```python
from build123d import *

# Parameters (mm, degrees)
BOSS_EXTRUDE1_DEPTH = 21
BOSS_EXTRUDE1_TAPER = 5
SKETCH2_R           = 1.5
CUT_EXTRUDE1_DEPTH  = 10
SKETCH3_R           = 2.75
CUT_EXTRUDE2_DEPTH  = 2


with BuildPart() as part:
    # Sketch1 → Boss-Extrude1 (new body)
    with BuildSketch(Plane.XY):
        with BuildLine():
            Line((-5.5, -7.5), (5.5, -7.5))
            ThreePointArc((5.5, -7.5), (6.914213562, -6.914213562), (7.5, -5.5))
            Line((7.5, -5.5), (7.5, 5.5))
            ThreePointArc((7.5, 5.5), (6.914213562, 6.914213562), (5.5, 7.5))
            Line((5.5, 7.5), (-5.5, 7.5))
            ThreePointArc((-5.5, 7.5), (-6.914213562, 6.914213562), (-7.5, 5.5))
            Line((-7.5, 5.5), (-7.5, -5.5))
            ThreePointArc((-7.5, -5.5), (-6.914213562, -6.914213562), (-5.5, -7.5))
        make_face()
    extrude(amount=BOSS_EXTRUDE1_DEPTH, taper=BOSS_EXTRUDE1_TAPER)

    # Sketch2 → Cut-Extrude1 (cut)
    with BuildSketch(Plane(origin=(0, 0, 0), x_dir=(-1, 0, 0), z_dir=(0, 0, -1))):
        Circle(SKETCH2_R)
    extrude(amount=-CUT_EXTRUDE1_DEPTH, mode=Mode.SUBTRACT)

    # Sketch3 → Cut-Extrude2 (cut)
    with BuildSketch(Plane.XY.offset(21)):
        Circle(SKETCH3_R)
    extrude(amount=-CUT_EXTRUDE2_DEPTH, mode=Mode.SUBTRACT)


solid = part.part
```
Geometry check sheet. Reference: the model listing, model coordinates, mm. A direction names the side the tool comes from. Coordinates: 2 decimals unless noted, no trailing zeros. Loops run counter-clockwise (first coordinate to the right, second up) from the corner with the lowest first, then second, coordinate; pieces in that order, holes last.
Item 1: Release check for a two-part mould opening along X. For faces 1 (the face through (6.594, 0.077, 10.353)), 2 (the face through (-0.596, -2.685, 20.014)), 3 (the face through (-6.26, -6.25, 10.65)) record: released by +X, released by -X, zero draft, split by the parting line, or undercut.
Item 2: Go/stop test with flat-tipped pins: pin 1 Ø2 at (x, z) = (-5, 18) entering from -Y; pin 2 Ø1.5 at (x, y) = (0, 0) entering from -Z; pin 3 Ø5 at (y, z) = (2, 13.5) entering from +X. Record where each tip stops, or that it passes through.
Item 3: Sectioned sample at B-B, the plane z = 9.25. Record the boundary of the cut face in (x, y).
Item 4: Sectioned sample at A-A, the plane x = 0. Record the boundary of the cut face in (y, z), then the cut area to 3 significant figures.
Item 5: Access from +Z, -Z, +X, -X, +Y, -Y to the whole of each face (thin tool, end or side, straight path). Record for faces 4 (the face through (-0.077, 6.594, 10.353)), 5 (the face through (1.5, 0.07, 4.93)), 6 (the face through (0, 0, 19)).
Item 6: Sectioned sample at D-D, the plane z = 11.75. Record the boundary of the cut face in (x, y), then the cut area to 3 significant figures.
Item 7: Thickness scan on line 1 (Y direction, x = 0, z = 3.25); line 2 (Z direction, x = 1.75, y = -1.5); line 3 (Y direction, x = 0, z = 19.8). Record the ranges inside material, lowest first.
Check result:
1. face 1: released by +X
1. face 2: undercut
1. face 3: released by -X
2. pin 1: stops at y = -6.01
2. pin 2: stops at z = 10
2. pin 3: stops at x = 6.54
3. outline: (-6.69, -5.5) arc R1.19 ccw to (-5.5, -6.69) - (5.5, -6.69) arc R1.19 ccw to (6.69, -5.5) - (6.69, 5.5) arc R1.19 ccw to (5.5, 6.69) - (-5.5, 6.69) arc R1.19 ccw to (-6.69, 5.5) - close; hole circle Ø3 at (0, 0)
4. outline: (-7.5, 0) - (-1.5, 0) - (-1.5, 10) - (1.5, 10) - (1.5, 0) - (7.5, 0) - (5.66, 21) - (2.75, 21) - (2.75, 19) - (-2.75, 19) - (-2.75, 21) - (-5.66, 21) - close
4. area: 235 mm2
5. face 4: +Z, +X, -X, +Y
5. face 5: -Z
5. face 6: +Z
6. outline: (-6.47, -5.5) arc R0.97 ccw to (-5.5, -6.47) - (5.5, -6.47) arc R0.97 ccw to (6.47, -5.5) - (6.47, 5.5) arc R0.97 ccw to (5.5, 6.47) - (-5.5, 6.47) arc R0.97 ccw to (-6.47, 5.5) - close
6. area: 167 mm2
7. line 1: y = -7.22 to -1.5, 1.5 to 7.22
7. line 2: z = 0 to 19
7. line 3: y = -5.77 to -2.75, 2.75 to 5.77
